Geometry: final body of the model. Coordinates: model frame, mm. Face numbers are marked on the shaded views. Give positions to 0.01 mm unless a question says otherwise; leave off trailing zeros. Order: outer loops, then holes, each group sorted by start corner. A loop starts at its lowest first (then second) coordinate and runs counter-clockwise, first axis right, second up. Notation, with made-up numbers: M 12,-23 L 45,-23 A13 cw 45,-19 Z; hole C 78,43.25 d9. An arc over 180 degrees is marked long. Use CSV: the item, a comma, the result in double quotes.
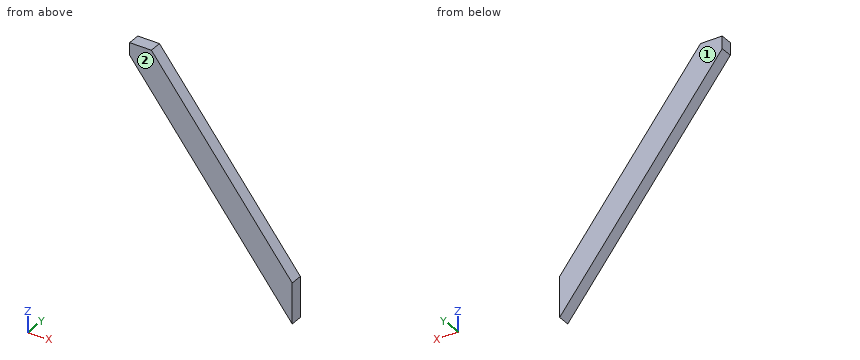
```python
from build123d import *

# Parameters (mm, degrees)
BOSS_EXTRUDE1_DEPTH = 50.8


with BuildPart() as part:
    # Sketch2 → Boss-Extrude1 (new body)
    with BuildSketch(Plane.XZ.offset(-710.7)):
        Polygon((665, 1298.940331748), (0, 2158.673017045), (0, 2209.8), (88.9, 2209.8), (665, 1465), align=None)
    extrude(amount=BOSS_EXTRUDE1_DEPTH)


solid = part.part
```
1. Pull-direction query (Y, two-part tool) for the marked faces 1 and 2; classes: +Y half, -Y half, draft (parallel to the pull), parting line (faces both ways), or undercut.
Answer:
face 1,"+Y half"
face 2,"-Y half"
2. Line query: line 1 (Z direction, x = 280, y = 699); line 2 (X direction, y = 691.5, z = 1730); line 3 (X direction, y = 704, z = 2065.5). Output: solid intervals per line, ascending.
Answer:
line 1,"1796.68 to 1962.74"
line 2,"331.58 to 460.02"
line 3,"72.07 to 200.52"
3. Section A-A, the plane y = 694.5. Return the cut outline in (x, z).
Answer:
outline,"M 0,2158.67 L 665,1298.94 L 665,1465 L 88.9,2209.8 L 0,2209.8 Z"
4. Pin query (flat end, axial travel): pin 1 Ø1 at (y, z) = (696.5, 2036) entering from +X; pin 2 Ø5 at (x, y) = (397, 693.5) entering from +Z; pin 3 Ø12 at (y, z) = (683.5, 1587) entering from +X. Return the tip coordinate at first contact, or that it passes through.
Answer:
pin 1,"x = 223.72"
pin 2,"z = 1814.71"
pin 3,"x = 575.27"
5. Section C-C, the plane x = 462. Return the cut outline in (y, z), plus the area to 3 significant figures.
Answer:
outline,"M 659.9,1561.39 L 710.7,1561.39 L 710.7,1727.44 L 659.9,1727.44 Z"
area,"8,440 mm2"
6. Section B-B, the plane z = 2046. Return the cut outline in (x, y).
Answer:
outline,"M 87.15,659.9 L 215.6,659.9 L 215.6,710.7 L 87.15,710.7 Z"
